Design review of the part shown in the three views and the two pictorial views. Dimensions are in mm from the part's minimum x, y and z. Coordinates: 2 decimals unless noted, no trailing zeros. Loops run counter-clockwise (first coordinate to the right, second up) from the corner with the lowest first, then second, coordinate; pieces in that order, holes last. Notation, with made-up numbers: (6, 56.25) -> (15, 56.25) arc R21 cw to (15, 95.25) -> close; hole circle Ø9 at (34.5, 2). An arc over 180 degrees is marked (long way). Answer in a Markdown table with one row per item.
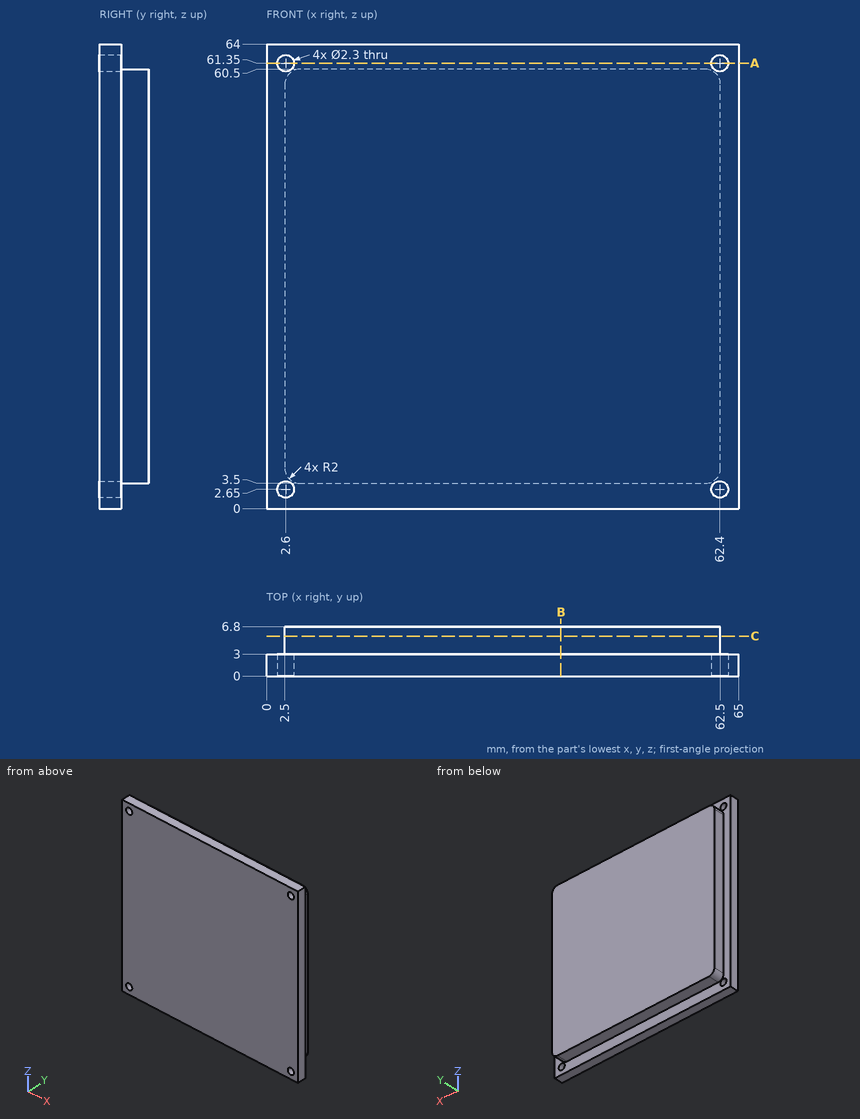
Item 1: Take a section at B-B, the plane x = 40.5. State the section outline as (y, z) points.
Worked answers:
| item | result |
|---|---|
| outline | (0, 0) -> (3, 0) -> (3, 3.5) -> (6.8, 3.5) -> (6.8, 60.5) -> (3, 60.5) -> (3, 64) -> (0, 64) -> close |
Item 2: Insertion check: pin 1 (1.9 mm diameter, centred on x = 21, y = 5, fed in from -Z); pin 2 (1.8 mm diameter, centred on x = 62.4, z = 2.65, fed in from +Y); pin 3 (2.5 mm diameter, centred on x = 2.6, z = 2.65, fed in from +Y); pin 4 (1.1 mm diameter, centred on y = 5, z = 36, fed in from +X). Each pin has a flat end and moves straight along its axis. Give the tip position at first contact, or say it passes through.
Worked answers:
| item | result |
|---|---|
| pin 1 | z = 3.5 |
| pin 2 | through |
| pin 3 | y = 3 |
| pin 4 | x = 62.5 |
Item 3: Take a section at C-C, the plane y = 5.5. State the section outline as (x, z) points, and give its area (3 significant figures).
Worked answers:
| item | result |
|---|---|
| outline | (2.5, 5.5) arc R2 ccw to (4.5, 3.5) -> (60.5, 3.5) arc R2 ccw to (62.5, 5.5) -> (62.5, 58.5) arc R2 ccw to (60.5, 60.5) -> (4.5, 60.5) arc R2 ccw to (2.5, 58.5) -> close |
| area | 3,420 mm² |
Item 4: For L1, parallel to X at y = 1.7, z = 2.65; L2, parallel to Z at x = 4.5, y = 4.5; L3, parallel to Y at x = 49, z = 61.5, list the stretches that pass through material, from the lowest coordinate up.
Worked answers:
| item | result |
|---|---|
| L1 | 0 to 1.45, 3.75 to 61.25, 63.55 to 65 |
| L2 | 3.5 to 60.5 |
| L3 | 0 to 3 |
Item 5: Take a section at A-A, the plane z = 61.35. State the section outline as (x, y) points, and give its area (3 significant figures).
Worked answers:
| item | result |
|---|---|
| outline | (0, 0) -> (1.45, 0) -> (1.45, 3) -> (0, 3) -> close; (3.75, 0) -> (61.25, 0) -> (61.25, 3) -> (3.75, 3) -> close; (63.55, 0) -> (65, 0) -> (65, 3) -> (63.55, 3) -> close |
| area | 181 mm² |
